from build123d import *

# Parameters (mm, degrees)
F0_W     = 408
F0_H     = 30
F1_DEPTH = 4


with BuildPart() as f1:
    # F0 (on Front) → F1 (new body)
    with BuildSketch(Plane.XZ):
        with Locations((0, 15)):
            Rectangle(F0_W, F0_H)
        with BuildLine():
            ThreePointArc((-177.5, 10), (-182.5, 15), (-177.5, 20))
            Line((-177.5, 20), (-107.5, 20))
            ThreePointArc((-107.5, 20), (-102.5, 15), (-107.5, 10))
            Line((-107.5, 10), (-177.5, 10))
        make_face(mode=Mode.SUBTRACT)
        with BuildLine():
            ThreePointArc((-82.5, 10), (-87.5, 15), (-82.5, 20))
            Line((-82.5, 20), (-12.5, 20))
            ThreePointArc((-12.5, 20), (-7.5, 15), (-12.5, 10))
            Line((-12.5, 10), (-82.5, 10))
        make_face(mode=Mode.SUBTRACT)
        with BuildLine():
            ThreePointArc((12.5, 10), (7.5, 15), (12.5, 20))
            Line((12.5, 20), (82.5, 20))
            ThreePointArc((82.5, 20), (87.5, 15), (82.5, 10))
            Line((82.5, 10), (12.5, 10))
        make_face(mode=Mode.SUBTRACT)
        with BuildLine():
            ThreePointArc((107.5, 10), (102.5, 15), (107.5, 20))
            Line((107.5, 20), (177.5, 20))
            ThreePointArc((177.5, 20), (182.5, 15), (177.5, 10))
            Line((177.5, 10), (107.5, 10))
        make_face(mode=Mode.SUBTRACT)
    extrude(amount=F1_DEPTH)


solid = f1.part
Build history of the part. All positions in model axes, mm. Coordinates: 2 decimals unless noted, no trailing zeros. Order: outer loops, then holes, each group sorted by start corner. A loop starts at its lowest first (then second) coordinate and runs counter-clockwise, first axis right, second up. Notation, with made-up numbers: M 80.5,65.5 L 101.5,65.5 A21 ccw 101.5,96.5 Z; hole C 67.5,37.25 d8. An arc over 180 degrees is marked long. One line per question, with ' | ' between items. Start each with the question number.
Q1. Probe L1, parallel to X at y = -1.4, z = 15; L2, parallel to Z at x = 168, y = -3.65; L3, parallel to X at y = -2.85, z = 15.75. List the from-to ranges inside material, lowest first. Write a range as from..to.
Q2. Saw through at A-A (y = -3.1). List the corners of the cut face in (x, z).
Q3. Saw through at B-B (x = -32.5). List the corners of the cut face in (y, z), then the cut area to 3 significant figures.
Check values:
1) L1: x = -204..-182.5, -102.5..-87.5, -7.5..7.5, 87.5..102.5, 182.5..204 | L2: z = 0..10, 20..30 | L3: x = -204..-182.44, -102.56..-87.44, -7.56..7.56, 87.44..102.56, 182.44..204
2) outline: M -204,0 L 204,0 L 204,30 L -204,30 Z; hole M -177.5,10 L -107.5,10 A5 ccw -107.5,20 L -177.5,20 A5 ccw Z; hole M -82.5,10 L -12.5,10 A5 ccw -12.5,20 L -82.5,20 A5 ccw Z; hole M 12.5,10 L 82.5,10 A5 ccw 82.5,20 L 12.5,20 A5 ccw Z; hole M 107.5,10 L 177.5,10 A5 ccw 177.5,20 L 107.5,20 A5 ccw Z
3) outline: M -4,0 L 0,0 L 0,10 L -4,10 Z; M -4,20 L 0,20 L 0,30 L -4,30 Z | area: 80.0 mm2
